The listing builds one solid part. Answer for the finished solid, in the listing's coordinates (mm). Coordinates: 2 decimals unless noted, no trailing zeros. Order: outer loops, then holes, each group sorted by start corner. A loop starts at its lowest first (then second) coordinate and runs counter-clockwise, first axis right, second up. Notation, with made-up numbers: (-15.75, 21) -> (10.25, 21) arc R21 ccw to (10.25, 33) -> close; hole circle Ø11 at (77, 40). An arc over 180 degrees is marked (long way). Answer in a Markdown table with one row per item.
```python
from build123d import *

# Parameters (mm, degrees)
F0_R   = 21.082
F0_R_2 = 17.526


with BuildPart() as f2:
    # F2: sweep along a path in F1
    with BuildLine(Plane.XZ) as f2_path:
        Line((0, 0), (0, 596.16388407))
        ThreePointArc((0, 596.16388407), (1.1576492205, 609.3958752082), (4.5954222961, 622.2258189914))
        Line((4.5954222961, 622.2258189914), (294.4944557647, 1418.7168673681))
        ThreePointArc((294.4944557647, 1418.7168673681), (322.3925090186, 1455.0743182215), (366.0990334686, 1468.8549324466))
        Line((366.0990334686, 1468.8549324466), (1681.7874046454, 1468.8549324466))
        ThreePointArc((1681.7874046454, 1468.8549324466), (1725.4939290954, 1455.0743182215), (1753.3919823493, 1418.7168673681))
        Line((1753.3919823493, 1418.7168673681), (2043.2910158179, 622.2258189914))
        ThreePointArc((2043.2910158179, 622.2258189914), (2046.7287888935, 609.3958752082), (2047.886438114, 596.16388407))
        Line((2047.886438114, 596.16388407), (2047.886438114, 0))
    # F0 (on Top) → F2 (sweep)
    with BuildSketch(Plane.XY):
        Circle(F0_R)
        Circle(F0_R_2, mode=Mode.SUBTRACT)
    sweep(path=f2_path.line)


solid = f2.part
```
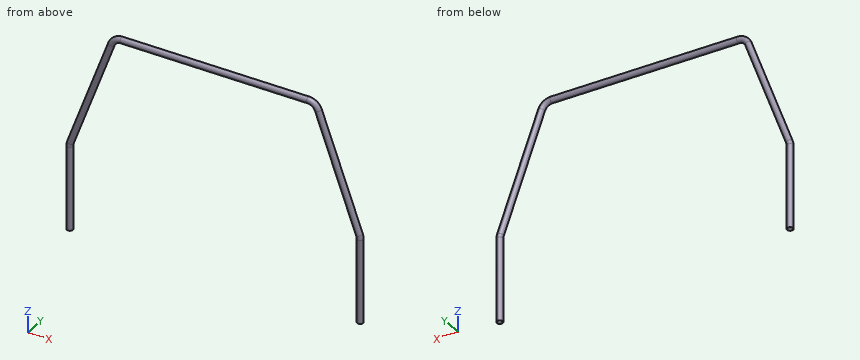
(1) A cutting plane is placed at A-A, the plane z = 165.5. Determine the outline of the cut face in (x, y).
Check values:
| item | result |
|---|---|
| outline | circle Ø42.16 at (0, 0); circle Ø42.16 at (2047.89, 0); hole circle Ø35.05 at (0, 0); hole circle Ø35.05 at (2047.89, 0) |
(2) A cutting plane is placed at C-C, the plane z = 1185. Count the separate pieces of the cut face and the enclosed holes in it, then the cut area to 3 significant figures.
Check values:
| item | result |
|---|---|
| separate pieces | 2 |
| enclosed holes | 2 |
| area | 918 mm² |
(3) Flat-ended cylindrical pins translate along their axes: pin 1 (4 mm diameter, centred on x = 674, y = 7.5, fed in from +Z); pin 2 (2 mm diameter, centred on y = -3, z = 581, fed in from -X); pin 3 (1 mm diameter, centred on y = 6.5, z = 160, fed in from +X). Find the tip coordinate at first contact, or state that the pin passes through.
Check values:
| item | result |
|---|---|
| pin 1 | z = 1489.21 |
| pin 2 | x = -20.99 |
| pin 3 | x = 2068.1 |
(4) Find the intervals of material crossed by line 1 along Z through (x, y) = (765, 3); line 2 along X through (y, z) = (5, 1087); line 3 along X through (y, z) = (-5, 1364), in increasing order. Write a range as from..to.
Check values:
| item | result |
|---|---|
| line 1 | 1447.99..1451.59, 1486.12..1489.72 |
| line 2 | 151.96..155.88, 191.64..195.55, 1852.33..1856.25, 1892..1895.92 |
| line 3 | 252.78..256.7, 292.45..296.37, 1751.51..1755.43, 1791.18..1795.1 |
(5) A cutting plane is placed at B-B, the plane x = 403. Determine the outline of the cut face in (y, z).
Check values:
| item | result |
|---|---|
| outline | circle Ø42.16 at (0, 1468.85); hole circle Ø35.05 at (0, 1468.85) |
